Geometry check sheet. Reference: the model listing, model coordinates, mm. Face numbers are marked on the shaded views. Coordinates: 2 decimals unless noted, no trailing zeros. Write each loop counter-clockwise with the first axis right and the second up, starting at its lowest first coordinate (ties: lowest second). Pieces come first, ordered by that corner, then holes. Notation, with made-up numbers: (-37.5, -30) -> (10.5, -30) arc R14 ccw to (10.5, -4) -> close; hole circle Ø9 at (83, 77.5). An arc over 180 degrees is marked (long way). Put each result on its own line as item: value. Start each with the question number.
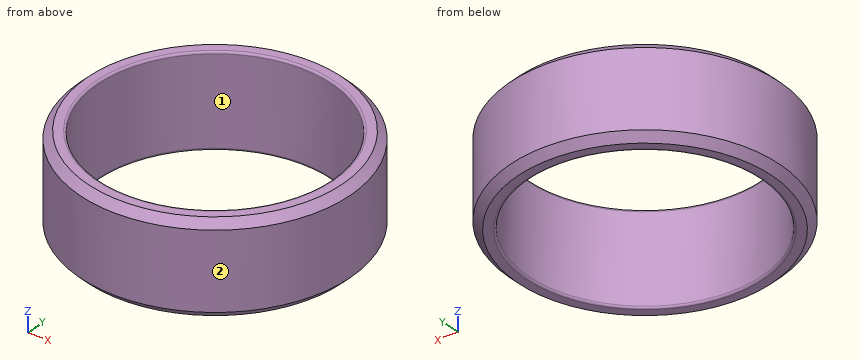
from build123d import *

# Parameters (mm, degrees)
F0_R     = 13.3
F0_R_2   = 11.5
F1_DEPTH = 9
F2_SIZE  = 0.75
F3_R     = 0.2
F4_R     = 0.2


with BuildPart() as f1:
    # F0 (on Top) → F1 (new body)
    with BuildSketch(Plane.XY):
        Circle(F0_R)
        Circle(F0_R_2, mode=Mode.SUBTRACT)
    extrude(amount=F1_DEPTH)

    # F2
    f2_edges = [f1.edges().sort_by_distance(p)[0] for p in [
        (-13.3, 0, 9),
        (-13.3, 0, 0),
    ]]
    chamfer(f2_edges, length=F2_SIZE)

    # F3
    f3_edges = [f1.edges().sort_by_distance(p)[0] for p in [
        (-11.5, 0, 9),
    ]]
    fillet(f3_edges, radius=F3_R)

    # F4
    f4_edges = [f1.edges().sort_by_distance(p)[0] for p in [
        (11.5, 0, 4.4),
        (-11.5, 0, 8.8),
        (-11.5, 0, 0),
    ]]
    fillet(f4_edges, radius=F4_R)


solid = f1.part
Item 1: Section check C-C, the plane z = 3.5. Enter the section's corners in (x, y), and give its area (3 significant figures).
Item 2: Mould release check, pull along X, two halves, no side actions. Record for the marked faces 1 and 2: released by +X, released by -X, zero draft, split by the parting line, or undercut.
Item 3: Go/stop test with flat-tipped pins: P1, Ø5, axis at y = -6.5, z = 5.5, coming from the -X side; P2, Ø5, axis at x = -10, z = 5.5, coming from the +Y side; P3, Ø14, axis at x = 0, y = 0, coming from the -Z side; P4, Ø1.5, axis at x = -5, z = 4.5, coming from the -Y side. Record where each tip stops, or that it passes through.
Item 4: Scan lines: line 1 along Y through (x, z) = (0, 4.5); line 2 along Y through (x, z) = (-6.25, 1.25); line 3 along Z through (x, y) = (6, 11.25). Record each from-to range of solid material in increasing order. Write a range as [from, to].
Item 5: Section check A-A, the plane y = 0. Enter the section's corners in (x, z).
From the geometry:
1. outline: circle Ø26.6 at (0, 0); hole circle Ø23 at (0, 0)
1. area: 140 mm²
2. face 1: undercut
2. face 2: split by the parting line
3. P1: x = -12.68
3. P2: y = 10.98
3. P3: through
3. P4: y = -12.6
4. line 1: [-13.3, -11.5], [11.5, 13.3]
4. line 2: [-11.74, -9.65], [9.65, 11.74]
4. line 3: [0.2, 8.8]
5. outline: (-13.3, 0.75) -> (-12.55, 0) -> (-11.7, 0) arc R0.2 ccw to (-11.5, 0.2) -> (-11.5, 8.8) arc R0.2 ccw to (-11.7, 9) -> (-12.55, 9) -> (-13.3, 8.25) -> close; (11.5, 0.2) arc R0.2 ccw to (11.7, 0) -> (12.55, 0) -> (13.3, 0.75) -> (13.3, 8.25) -> (12.55, 9) -> (11.7, 9) arc R0.2 ccw to (11.5, 8.8) -> close
